from build123d import *

# Parameters (mm, degrees)
F0_R     = 2.9972
F1_DEPTH = 5.842
F0_R_2   = 4.0005
F2_DEPTH = 1.651
F3_R     = 2.027538
F4_DEPTH = 25.4


with BuildPart() as f1:
    # F0 (on Front) → F1 (new body)
    with BuildSketch(Plane.XZ):
        Circle(F0_R)
    extrude(amount=F1_DEPTH)

    # F0 (on Front) → F2 (join)
    with BuildSketch(Plane.XZ):
        Circle(F0_R_2)
        Circle(F0_R, mode=Mode.SUBTRACT)
    extrude(amount=F2_DEPTH)

    # F3 (on Front) → F4 (join)
    with BuildSketch(Plane.XZ):
        Circle(F3_R)
    extrude(amount=F4_DEPTH)


solid = f1.part
Model file for the job. Use its own axes, mm. A direction names the side the tool comes from. Give positions to 0.01 mm unless a question says otherwise; leave off trailing zeros. Order: outer loops, then holes, each group sorted by start corner. A loop starts at its lowest first (then second) coordinate and runs counter-clockwise, first axis right, second up. Notation, with made-up numbers: (86, 89) - (106, 89) arc R23 cw to (106, 128) - close; hole circle Ø11 at (4.25, -29.5). An arc over 180 degrees is marked (long way). One line per item, written item: value.
Item 1: Pin check, flat tips, straight feed: pin 1 Ø4 at (y, z) = (-6.5, 1) entering from +X; pin 2 Ø2 at (x, y) = (0.5, -18.5) entering from +Z; pin 3 Ø1 at (x, y) = (-2, -5) entering from -Z. Stop position of each tip, or through.
Response values:
pin 1: x = 3
pin 2: z = 2.03
pin 3: z = -2.59
Item 2: Two-plate mould, pull along Y, no slides. Class faces 1 (the cylindrical face through (-0.9, -0.8, -3.9)), 2 (the flat face through (1, -1.651, 3)), 3 (the flat face through (0, 0, 0)): released by +Y, released by -Y, zero draft, split by the parting line, or undercut.
Response values:
face 1: zero draft
face 2: released by -Y
face 3: released by +Y
Item 3: Tool access for faces 4 (the flat face through (0, -25.4, 0)), 5 (the cylindrical face through (2.86, -3.72, 0.9)): list every direction of +Z, -Z, +X, -X, +Y, -Y with a clear straight run to the whole face (end or side of a thin tool).
Response values:
face 4: +Z, -Z, +X, -X, -Y
face 5: -Y
Item 4: Slice it at A-A (x = 0). List the corners of the cut face in (y, z), then the cut area to 3 significant figures.
Response values:
outline: (-25.4, -2.03) - (-5.84, -2.03) - (-5.84, -3) - (-1.65, -3) - (-1.65, -4) - (0, -4) - (0, 4) - (-1.65, 4) - (-1.65, 3) - (-5.84, 3) - (-5.84, 2.03) - (-25.4, 2.03) - close
area: 118 mm2
Item 5: Slice it at C-C (y = -16.5). List the corners of the cut face in (x, z), then the cut area to 3 significant figures.
Response values:
outline: circle Ø4.06 at (0, 0)
area: 12.9 mm2
Item 6: Slice it at D-D (x = -2.5). List the corners of the cut face in (y, z).
Response values:
outline: (-5.84, -1.65) - (-1.65, -1.65) - (-1.65, -3.12) - (0, -3.12) - (0, 3.12) - (-1.65, 3.12) - (-1.65, 1.65) - (-5.84, 1.65) - close
Item 7: Wall check: line 1 (Y direction, x = 2, z = -1.75); line 2 (Z direction, x = 0, y = -4.75); line 3 (Y direction, x = -1.5, z = 2.75). Give the ranges that are in metal, low to high.
Response values:
line 1: -5.84 to 0
line 2: -3 to 3
line 3: -1.65 to 0
Item 8: Slice it at B-B (z = 0). List the corners of the cut face in (x, y), then the cut area to 3 significant figures.
Response values:
outline: (-4, -1.65) - (-3, -1.65) - (-3, -5.84) - (-2.03, -5.84) - (-2.03, -25.4) - (2.03, -25.4) - (2.03, -5.84) - (3, -5.84) - (3, -1.65) - (4, -1.65) - (4, 0) - (-4, 0) - close
area: 118 mm2
